The listing builds one solid part. Answer for the finished solid, in the listing's coordinates (mm). A direction names the side the tool comes from. Round coordinates to 2 decimals unless told otherwise and drop trailing zeros. Loops run counter-clockwise (first coordinate to the right, second up) from the corner with the lowest first, then second, coordinate; pieces in that order, holes last. Notation, with made-up numbers: (10.25, 53) -> (17.25, 53) arc R16 cw to (17.25, 57) -> close; hole circle Ø2 at (11.5, -7). An arc over 180 degrees is marked (long way). Use a Markdown table: item, result. Add a question column.
Q1. Section B-B on x = 50 is taken. Give the vertices of the cut face in (y, z).
Q2. Section A-A on y = 52.5 is taken. Give the vertices of the cut face in (x, z).
Q3. Which of the six approach directions +Z, -Z, +X, -X, +Y, -Y give full straight-line access (tool end or side, diameter ignored) to faces 1 (the flat face through (40, 41, 0)), 2 (the cylindrical face through (-0.683, 40.56, -1.73))?
Q4. Given pin 1 Ø1 at (y, z) = (69.5, 0) entering from -X, flat-ended and moving along its own axis, determine where the tip first touches the part or whether it passes through.
Q5. Consider line 1 (X direction, y = 39, z = -1); line 2 (Z direction, x = 7, y = 56); line 3 (X direction, y = 59, z = -0.7). Determine where each line is inside the solid, lowest interval first.
from build123d import *

# Parameters (mm, degrees)
ESQUISSE1_W        = 80
ESQUISSE1_H        = 80
BOSS_EXTRU_1_DEPTH = 1
ESQUISSE2_R        = 0.5
BOSS_EXTRU_2_DEPTH = 80


with BuildPart() as part:
    # Esquisse1 → Boss.-Extru.1 (new body)
    with BuildSketch(Plane.XY):
        with Locations((40, 40)):
            Rectangle(ESQUISSE1_W, ESQUISSE1_H)
    extrude(amount=BOSS_EXTRU_1_DEPTH)

    # Esquisse2 → Boss.-Extru.2 (add)
    with BuildSketch(Plane(origin=(0, 80, 0), x_dir=(1, 0, 0), z_dir=(0, 1, 0))):
        with BuildLine():
            Line((1, 0), (1, 1))
            ThreePointArc((1, 1), (-0.707106781, 1.707106781), (0, 0))
            Line((0, 0), (1, 0))
        make_face()
        with Locations(Location((0, 1, 0), (0, 0, 270))):
            Circle(ESQUISSE2_R, mode=Mode.SUBTRACT)
    extrude(amount=-BOSS_EXTRU_2_DEPTH)


solid = part.part
Checked values:
| question | item | result |
|---|---|---|
| 1 | outline | (0, 0) -> (80, 0) -> (80, 1) -> (0, 1) -> close |
| 2 | outline | (0, 0) arc R1 ccw (long way) to (1, -1) -> (1, 0) -> (80, 0) -> (80, 1) -> (0, 1) -> close; hole circle Ø1 at (0, -1) |
| 3 | face 1 | -Z, +X, +Y, -Y |
| 3 | face 2 | +Y, -Y |
| 4 | pin 1 | stops at x = -0.87 |
| 5 | line 1 | x = -1 to -0.5, 0.5 to 1 |
| 5 | line 2 | z = 0 to 1 |
| 5 | line 3 | x = -0.95 to -0.4, 0.4 to 1 |
